Geometry check sheet. Reference: the model listing, model coordinates, mm. Face numbers are marked on the shaded views. A direction names the side the tool comes from. Give positions to 0.01 mm unless a question says otherwise; leave off trailing zeros. Order: outer loops, then holes, each group sorted by start corner. A loop starts at its lowest first (then second) coordinate and runs counter-clockwise, first axis right, second up.
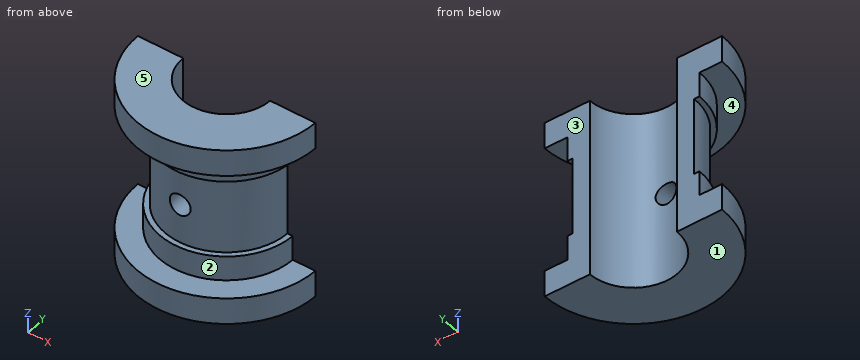
from build123d import *

# Parameters (mm, degrees)
REVOLVE1_ANGLE     = 180
SKETCH2_R          = 3
CUT_EXTRUDE1_DEPTH = 18.5


with BuildPart() as part:
    # Sketch1 → Revolve1 (revolve)
    with BuildSketch(Plane(origin=(0, 0, 0), x_dir=(1, 0, 0), z_dir=(0, 1, 0))):
        Polygon((-25.5, 25.5), (-25.5, 18), (-19, 18), (-19, 11), (-17.5, 11), (-17.5, -11), (-19, -11), (-19, -18), (-25.5, -18), (-25.5, -25.5), (-12.5, -25.5), (-12.5, 25.5), align=None)
    revolve(axis=Axis((0, 0, 0), (0, 0, 1)), revolution_arc=REVOLVE1_ANGLE)

    # Sketch2 → Cut-Extrude1 (cut, through all)
    with BuildSketch(Plane(origin=(0, -17.5, 0), x_dir=(-1, 0, 0), z_dir=(0, -1, 0))):
        with Locations(Location((0, 0, 0), (0, 0, 90))):  # turned: the seam where the file's is
            Circle(SKETCH2_R)
    extrude(amount=-CUT_EXTRUDE1_DEPTH, mode=Mode.SUBTRACT)


solid = part.part
Item 1: Gauge pin test, flat ends, axial feed: pin 1 (7 mm diameter, centred on x = 0, z = 0, fed in from -Y); pin 2 (15 mm diameter, centred on x = 8, y = -9.5, fed in from -Z); pin 3 (3 mm diameter, centred on y = -16.5, z = -6.5, fed in from -X); pin 4 (4 mm diameter, centred on y = -18, z = 4, fed in from +X). Record the tip position at first contact, or that the pin passes through.
Reported:
pin 1: stops at y = -17.5
pin 2: stops at z = -25.5
pin 3: stops at x = -9.01
pin 4: stops at x = 7.09
Item 2: Sectioned sample at A-A (x = 0). Enter the section's corners in (y, z), and give its area (3 significant figures).
Reported:
outline: (-25.5, -25.5) - (-12.5, -25.5) - (-12.5, -3) - (-17.5, -3) - (-17.5, -11) - (-19, -11) - (-19, -18) - (-25.5, -18) - close; (-25.5, 18) - (-19, 18) - (-19, 11) - (-17.5, 11) - (-17.5, 3) - (-12.5, 3) - (-12.5, 25.5) - (-25.5, 25.5) - close
area: 366 mm2
Item 3: Sectioned sample at C-C (z = 0). Enter the section's corners in (x, y).
Reported:
outline: (-17.5, 0) arc R17.5 ccw to (-3, -17.24) - (-3, -12.13) arc R12.5 cw to (-12.5, 0) - close; (3, -17.24) arc R17.5 ccw to (17.5, 0) - (12.5, 0) arc R12.5 cw to (3, -12.13) - close
Item 4: Draft check along Z on the marked faces 1, 2 and 3. Enter one of: released by +Z, released by -Z, zero draft, split by the parting line, or undercut.
Reported:
face 1: released by -Z
face 2: undercut
face 3: zero draft
Item 5: Set-up check for the marked faces 4 and 5: record each of +Z, -Z, +X, -X, +Y, -Y from which the full face is reachable in a straight line by a thin tool's end or side.
Reported:
face 4: -Y
face 5: +Z, +X, -X, +Y, -Y
Item 6: Sectioned sample at D-D (z = -8). Enter the section's corners in (x, y).
Reported:
outline: (-17.5, 0) arc R17.5 ccw to (17.5, 0) - (12.5, 0) arc R12.5 cw to (-12.5, 0) - close
Item 7: Scan lines: L1, parallel to Z at x = 0, y = -16.2; L2, parallel to Z at x = -20.5, y = -5.75; L3, parallel to Y at x = -0.5, z = -21.5. Record each from-to range of solid material in increasing order.
Reported:
L1: z = -25.5 to -3, 3 to 25.5
L2: z = -25.5 to -18, 18 to 25.5
L3: y = -25.5 to -12.49
Item 8: Sectioned sample at B-B (y = -5.75). Enter the section's corners in (x, z), and give its area (3 significant figures).
Reported:
outline: (-24.84, -25.5) - (-11.1, -25.5) - (-11.1, 25.5) - (-24.84, 25.5) - (-24.84, 18) - (-18.11, 18) - (-18.11, 11) - (-16.53, 11) - (-16.53, -11) - (-18.11, -11) - (-18.11, -18) - (-24.84, -18) - close; (11.1, -25.5) - (24.84, -25.5) - (24.84, -18) - (18.11, -18) - (18.11, -11) - (16.53, -11) - (16.53, 11) - (18.11, 11) - (18.11, 18) - (24.84, 18) - (24.84, 25.5) - (11.1, 25.5) - close
area: 848 mm2
